The model under review builds one solid part; all positions refer to its coordinate system, in mm. A direction names the side the tool comes from. Round coordinates to 2 decimals unless told otherwise and drop trailing zeros. Write each loop counter-clockwise with the first axis right and the second up, starting at its lowest first coordinate (ties: lowest second). Pieces come first, ordered by that corner, then holes.
Item 1: Add section A-A (y = 46.5). Give the boundary of the cut face in (x, z), plus the area to 3 significant figures.
Item 2: Add section C-C (x = 65). Give the boundary of the cut face in (y, z).
Item 3: Draft analysis for pull direction Z (two halves, no side actions). For faces 4 (the face through (65, 40, 23)), 5 (the face through (25, 20, 15)), 6 (the face through (48, 19, 30)), state which applies: +Z half, -Z half, draft (parallel to the pull), parting line (faces both ways), or undercut.
Item 4: Clearance check with flat-ended pins moving along their axes: pin 1 Ø5 at (y, z) = (23, 27) entering from -X; pin 2 Ø2.5 at (x, z) = (64.5, 6.5) entering from +Y; pin 3 Ø2.5 at (x, z) = (64, 24) entering from +Y; pin 4 Ø3 at (x, z) = (29, 3) entering from +Y. State where each tip first meets the part, or that it passes through.
Item 5: Add section B-B (z = 7). Give the boundary of the cut face in (x, y).
Item 6: Machinability: for faces 1 (the face through (80, 25, 15)), 2 (the face through (50, 35, 15)), 3 (the face through (65.1, 45.1, 20.5)), which of the approach directions +Z, -Z, +X, -X, +Y, -Y give a long, thin tool a straight path to every point of the face, cutting with its end or side? Answer none if there is none.
Item 7: To check wall thickness, follow L1, parallel to X at y = 42.5, z = 23; L2, parallel to X at y = 29.5, z = 1; L3, parallel to Y at x = 30.5, z = 1.5. State the ranges of each line that lie inside material, in increasing order.
Item 8: Add section D-D (y = 26). Give the boundary of the cut face in (x, z).
```python
from build123d import *

# Parameters (mm, degrees)
SKETCH1_W           = 80
SKETCH1_H           = 20
BOSS_EXTRUDE1_DEPTH = 30
SKETCH13_W          = 30
SKETCH13_H          = 30
BOSS_EXTRUDE7_DEPTH = 30
SKETCH14_R          = 2.5
CUT_EXTRUDE1_DEPTH  = 10


with BuildPart() as part:
    # Sketch1 → Boss-Extrude1 (new body)
    with BuildSketch(Plane.XY):
        with Locations((40, 10)):
            Rectangle(SKETCH1_W, SKETCH1_H)
    extrude(amount=BOSS_EXTRUDE1_DEPTH)

    # Sketch13 → Boss-Extrude7 (add)
    with BuildSketch(Plane(origin=(0, 20, 0), x_dir=(1, 0, 0), z_dir=(0, 1, 0))):
        with Locations((65, -15)):
            Rectangle(SKETCH13_W, SKETCH13_H)
    extrude(amount=BOSS_EXTRUDE7_DEPTH)

    # Sketch14 → Cut-Extrude1 (cut)
    with BuildSketch(Plane(origin=(0, 50, 0), x_dir=(1, 0, 0), z_dir=(0, 1, 0))):
        with Locations(Location((65, -7, 0), (0, 0, 270))):
            Circle(SKETCH14_R)
        with Locations(Location((65, -23, 0), (0, 0, 270))):
            Circle(SKETCH14_R)
    extrude(amount=-CUT_EXTRUDE1_DEPTH, mode=Mode.SUBTRACT)


solid = part.part
```
Numbers:
1. outline: (50, 0) - (80, 0) - (80, 30) - (50, 30) - close; hole circle Ø5 at (65, 7); hole circle Ø5 at (65, 23)
1. area: 861 mm2
2. outline: (0, 0) - (50, 0) - (50, 4.5) - (40, 4.5) - (40, 9.5) - (50, 9.5) - (50, 20.5) - (40, 20.5) - (40, 25.5) - (50, 25.5) - (50, 30) - (0, 30) - close
3. face 4: undercut
3. face 5: draft
3. face 6: +Z half
4. pin 1: stops at x = 50
4. pin 2: stops at y = 40
4. pin 3: stops at y = 50
4. pin 4: stops at y = 20
5. outline: (0, 0) - (80, 0) - (80, 50) - (67.5, 50) - (67.5, 40) - (62.5, 40) - (62.5, 50) - (50, 50) - (50, 20) - (0, 20) - close
6. face 1: +Z, -Z, +X, +Y, -Y
6. face 2: +Z, -Z, -X, +Y
6. face 3: +Y
7. L1: x = 50 to 62.5, 67.5 to 80
7. L2: x = 50 to 80
7. L3: y = 0 to 20
8. outline: (50, 0) - (80, 0) - (80, 30) - (50, 30) - close
